```python
from build123d import *

# Parameters (mm, degrees)
F1_DEPTH = 22.352
F2_DEPTH = 3.175
F4_R     = 22.35199
F5_DEPTH = 25.4
F6_R     = 3.175
F7_DEPTH = 25.4
F8_R     = 6.35
F8_R_2   = 3.175
F9_DEPTH = 3.175
F10_R    = 10.922


# Not quite as in the source:
# - a fillet or chamfer is up to 0.001 mm smaller than in the source, because OpenCascade refuses the exact size


with BuildPart() as f1:
    # F0 (on Front) → F1 (new body, symmetric)
    with BuildSketch(Plane.XZ):
        Polygon((0, 0), (-25.4, 0), (-44.45, 32.9955678842), (-52.7857543947, 28.1829178405), (-30.9417543947, -9.652), (60.452, -9.652), (60.452, 0), align=None)
    extrude(amount=F1_DEPTH, both=True)

    # F0 (on Front) → F2 (join, symmetric)
    with BuildSketch(Plane.XZ):
        Polygon((-44.45, 32.9955678842), (-25.4, 0), (0, 0), align=None)
    extrude(amount=F2_DEPTH, both=True)

    # F4 (radius 22.352 in the source; OpenCascade refuses exactly that, so slightly less here)
    f4_edges = [f1.edges().sort_by_distance(p)[0] for p in [
        (60.452, -22.352, -4.826),
        (60.452, 22.352, -4.826),
    ]]
    fillet(f4_edges, radius=F4_R)

    # F3 (on face) → F5 (cut)
    with BuildSketch(Plane.XY):
        with BuildLine():
            ThreePointArc((12.7, 9.652), (3.048, 0), (12.7, -9.652))
            Line((12.7, -9.652), (40.1388603866, -9.652))
            ThreePointArc((40.1388603866, -9.652), (49.7908603866, 0), (40.1388603866, 9.652))
            Line((40.1388603866, 9.652), (12.7, 9.652))
        make_face()
    extrude(amount=-F5_DEPTH, mode=Mode.SUBTRACT)

    # F6 (on face) → F7 (cut)
    with BuildSketch(Plane(origin=(-27.3857543947, 0, -15.8111726717), x_dir=(0, -1, 0), z_dir=(-0.8660254038, 0, -0.5))):
        with Locations((11.8134439608, 39.878)):
            Circle(F6_R)
        with Locations((-11.43, 39.878)):
            Circle(F6_R)
    extrude(amount=-F7_DEPTH, mode=Mode.SUBTRACT)

    # F8 (on face) → F9 (cut)
    with BuildSketch(Plane(origin=(-19.05, 0, -10.9985226281), x_dir=(0, 1, 0), z_dir=(0.8660254038, 0, 0.5))):
        with Locations((-11.8134439608, 39.878)):
            Circle(F8_R)
        with Locations((-11.8134439608, 39.878)):
            Circle(F8_R_2, mode=Mode.SUBTRACT)
        with Locations((11.43, 39.878)):
            Circle(F8_R)
    extrude(amount=-F9_DEPTH, mode=Mode.SUBTRACT)

    # F10
    f10_edges = [f1.edges().sort_by_distance(p)[0] for p in [
        (-48.617877, -22.352, 30.589243),
        (-48.617877, 22.352, 30.589243),
    ]]
    fillet(f10_edges, radius=F10_R)


solid = f1.part
```
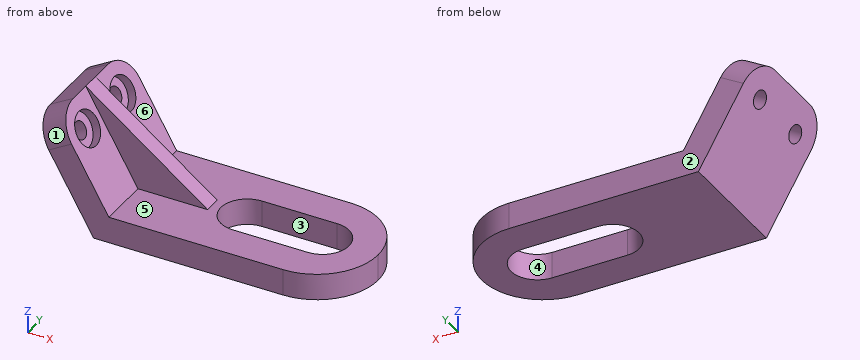
For this review, take the finished solid that the model builds, in its own axes (mm). Face numbers are marked on the shaded views. A direction names the side the tool comes from. Round coordinates to 2 decimals unless told otherwise and drop trailing zeros. Write each loop counter-clockwise with the first axis right and the second up, starting at its lowest first coordinate (ties: lowest second). Pieces come first, ordered by that corner, then holes. Notation, with made-up numbers: (21, 54) - (48, 54) arc R18 cw to (48, 62) - close; hole circle Ø9 at (55, -7). An arc over 180 degrees is marked (long way). Put each result on its own line as item: value.
Q1. Mouldability with a two-part tool opening along Y and no side actions: class the marked faces 1, 2 and 3 as released by +Y, released by -Y, zero draft, split by the parting line, or undercut.
Solved:
face 1: released by -Y
face 2: released by +Y
face 3: undercut
Q2. Machinability: for the marked faces 4, 5 and 6, which of the approach directions +Z, -Z, +X, -X, +Y, -Y give a long, thin tool a straight path to every point of the face, cutting with its end or side? Answer none if there is none.
Solved:
face 4: +Z, -Z
face 5: +Z, +X
face 6: +Z, +X, +Y
Q3. We need section B-B (y = -7.5). Give the boundary of the cut face in (x, z), and give its area (3 significant figures).
Solved:
outline: (-52.79, 28.18) - (-30.94, -9.65) - (6.62, -9.65) - (6.62, 0) - (-25.4, 0) - (-36.66, 19.5) - (-39.41, 17.91) - (-44.07, 25.99) - (-41.32, 27.57) - (-44.45, 33) - close; (46.21, -9.65) - (59.16, -9.65) - (59.16, 0) - (46.21, 0) - close
area: 825 mm2
Q4. We need section A-A (x = 29). Give the boundary of the cut face in (y, z).
Solved:
outline: (-22.35, -9.65) - (-9.65, -9.65) - (-9.65, 0) - (-22.35, 0) - close; (9.65, -9.65) - (22.35, -9.65) - (22.35, 0) - (9.65, 0) - close
Q5. We need section D-D (x = -8.5). Give the boundary of the cut face in (y, z) (3 decimals).
Solved:
outline: (-22.352, -9.652) - (22.352, -9.652) - (22.352, 0) - (3.175, 0) - (3.175, 6.31) - (-3.175, 6.31) - (-3.175, 0) - (-22.352, 0) - close
Q6. Wall thickness on probe 1 along Y at (x, z) = (13.5, -7); probe 2 along Z at (x, y) = (9, -12); probe 3 along Y at (x, z) = (-43, 20): over which ranges is each line inside the solid? List them lowest first.
Solved:
probe 1: y = -22.35 to -9.65, 9.65 to 22.35
probe 2: z = -9.65 to 0
probe 3: y = -22.35 to -14.81, -8.82 to 8.44, 14.42 to 22.35
Q7. Insertion check: pin 1 Ø16.5 at (x, z) = (-19, 13.5) entering from +Y (3 decimals); pin 2 Ø3 at (x, y) = (0.5, -16) entering from +Z; pin 3 Ø2 at (y, z) = (-13.5, 16.5) entering from +X. Each pin has a flat end and moves straight along its axis. Give the tip position at first contact, or say it passes through.
Solved:
pin 1: stops at y = 3.175
pin 2: stops at z = 0
pin 3: stops at x = -34.35
Q8. We need section C-C (z = 13.5). Give the boundary of the cut face in (x, y) (3 decimals), and give its area (3 significant figures).
Solved:
outline: (-44.309, -22.352) - (-33.194, -22.352) - (-33.194, -3.175) - (-18.187, -3.175) - (-18.187, 3.175) - (-33.194, 3.175) - (-33.194, 22.352) - (-44.309, 22.352) - close
area: 592 mm2
